Autodesk Inventor part; units mm, degrees
ref_plane "YZ Plane" through (0, 0, 0) normal (1, 0, 0) x (0, 1, 0)
ref_plane "XZ Plane" through (0, 0, 0) normal (0, 1, 0) x (-1, 0, 0)
ref_plane "XY Plane" through (0, 0, 0) normal (0, 0, 1) x (1, 0, 0)
sketch "Sketch1" plane through (0, 0, 0) normal (0, 0, 1) x (1, 0, 0)
  line L0 (-60, -20) -> (60, -20)
  line L1 (60, -20) -> (60, 20)
  line L2 (60, 20) -> (-60, 20)
  line L3 (-60, 20) -> (-60, -20)
  line L4 (-60, -20) -> (60, 20) construction
  line L5 (60, -20) -> (-60, 20) construction
  circle A0 centre (28.637, -15.621) radius 1.5875
  circle A1 centre (9.587, -15.621) radius 1.5875
  circle A2 centre (-9.463, -15.621) radius 1.5875
  circle A3 centre (28.637, 15.621) radius 1.5875
  circle A4 centre (9.587, 15.621) radius 1.5875
  circle A5 centre (-9.463, 15.621) radius 1.5875
  circle A6 centre (50, -10) radius 2.5
  circle A7 centre (50, 10) radius 2.5
  circle A8 centre (-50, -10) radius 2.5
  circle A9 centre (-50, 10) radius 2.5
  point P0 (0, 0)
  dimension "d0" = 120
  dimension "d1" = 40
  dimension "d4" = 3.175
  dimension "d5" = 3.175
  dimension "d6" = 3.175
  dimension "d7" = 3.175
  dimension "d8" = 3.175
  dimension "d9" = 3.175
  dimension "d10" = 31.242
  dimension "d11" = 19.05
  dimension "d12" = 19.05
  dimension "d13" = 31.363
  dimension "d14" = 5
  dimension "d15" = 5
  dimension "d16" = 5
  dimension "d17" = 5
  dimension "d20" = 10
  dimension "d21" = 10
  dimension "d22" = 20
  dimension "d23" = 10
  dimension "d26" = 4.379
extrude "Extrusion2" add sketch "Sketch1" along normal mid plane 6
properties part number "motor_bracket_base"
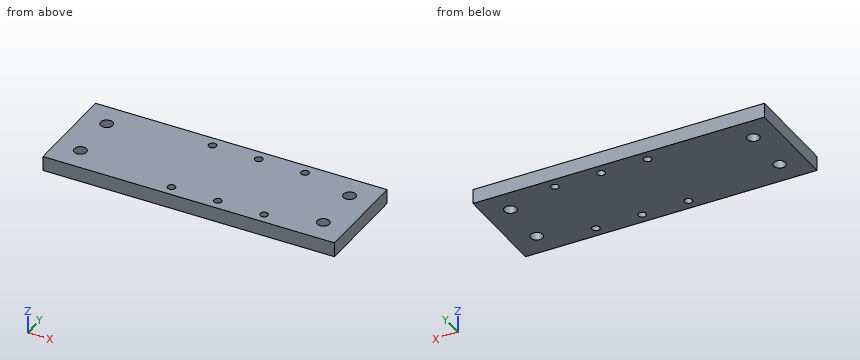
Geometry: final body of the model. Coordinates: model frame, mm. Coordinates: 2 decimals unless noted, no trailing zeros. Order: outer loops, then holes, each group sorted by start corner. A loop starts at its lowest first (then second) coordinate and runs counter-clockwise, first axis right, second up.
1) Section A-A (y = -10). Return loops of the section in (x, z).
Result sheet:
outline: (-60, -3) - (-52.5, -3) - (-52.5, 3) - (-60, 3) - close; (-47.5, -3) - (47.5, -3) - (47.5, 3) - (-47.5, 3) - close; (52.5, -3) - (60, -3) - (60, 3) - (52.5, 3) - close
2) Ray query, probe 1 along Y at (x, z) = (-50, -0.9); probe 2 along Y at (x, z) = (9.5, 1.25); probe 3 along X at (y, z) = (15, 2). Return the intervals inside material, ascending.
Result sheet:
probe 1: y = -20 to -12.5, -7.5 to 7.5, 12.5 to 20
probe 2: y = -20 to -17.21, -14.04 to 14.04, 17.21 to 20
probe 3: x = -60 to -10.92, -8 to 8.13, 11.05 to 27.18, 30.1 to 60
3) First-contact query: P1, Ø3, axis at x = 50, y = 10, coming from the -Z side. Flat tip, straight axial feed; report the tip coordinate or a pass-through.
Result sheet:
P1: passes through
4) Section C-C (z = -1). Give the number of separate pieces and of enclosed holes in the cut face, then the cut area to 3 significant figures.
Result sheet:
separate pieces: 1
enclosed holes: 10
area: 4,670 mm2
5) Section B-B (x = -50). Return loops of the section in (y, z).
Result sheet:
outline: (-20, -3) - (-12.5, -3) - (-12.5, 3) - (-20, 3) - close; (-7.5, -3) - (7.5, -3) - (7.5, 3) - (-7.5, 3) - close; (12.5, -3) - (20, -3) - (20, 3) - (12.5, 3) - close
